Here's how the part is built. I have some questions about the finished solid (model axes, mm). A direction names the side the tool comes from. Coordinates: 2 decimals unless noted, no trailing zeros. Loops run counter-clockwise (first coordinate to the right, second up) from the corner with the lowest first, then second, coordinate; pieces in that order, holes last. Notation, with made-up numbers: (-23, 43.5) -> (-18, 43.5) arc R15 cw to (-18, 71.5) -> close; hole circle Ø5 at (6, 71.25). An arc over 180 degrees is marked (long way). Answer as a JSON object with one key per item and string values. Group by question number.
Q1. I want a section at A-A on z = -129. Write out the boundary of the cut face in (x, y).
Q2. I'm going to push flat-ended pins straight in: pin 1 (2 mm diameter, centred on x = -23, z = -92.5, fed in from -Y); pin 2 (12 mm diameter, centred on y = 8, z = -45, fed in from -X); pin 3 (1 mm diameter, centred on x = 4, z = -14.5, fed in from -Y). Where does each tip first touch, or does it pass through?
Q3. I need wall thicknesses on line 1 (Z direction, x = 36.5, y = 57); line 2 (Z direction, x = -36, y = 43.5); line 3 (X direction, y = -35, z = -122). Which ranges of each line are inside material? Lowest first, please.
Q4. I want a section at B-B on z = -12. Write out the boundary of the cut face in (x, y).
Q5. Thinking about a two-plate mould opening in Y: for faces 3 (the flat face through (0, 0, 47.5)), 4 (the conical face through (6.068, 46.217, -59.383)), which applies, released by +Y, released by -Y, zero draft, split by the parting line, or undercut?
Q6. On a 3-axis mill with a long thin cutter (end or side, diameter ignored), from which of +Z, -Z, +X, -X, +Y, -Y can I reach the whole of each face in a straight line? I mean faces 1 (the flat face through (1, 1, -150)), 2 (the cylindrical face through (12.365, -19.394, 3.014)). Say none if no direction works.
```python
from build123d import *

# Parameters (mm, degrees)
FILLET1_R = 10


with BuildPart() as part:
    # Sketch1 → Revolve1 (revolve)
    with BuildSketch(Plane.YZ, mode=Mode.PRIVATE) as revolve1_sk:
        with BuildLine():
            Line((0, 0), (-25, 0))
            Line((-25, 0), (-25, 2))
            Line((-25, 2), (-23, 2))
            Line((-23, 2), (-23, 4))
            ThreePointArc((-23, 4), (-19.907119135, 18.74298562), (-11.15, 31))
            Line((-11.15, 31), (-11.15, 47.5))
            Line((-11.15, 47.5), (0, 47.5))
            Line((0, 47.5), (0, 0))
        make_face()
    revolve(revolve1_sk.sketch.rotate(Axis((0, 0, 47.5), (0, 0, -1)), 270), axis=Axis((0, 0, 47.5), (0, 0, -1)))

    # Fillet1
    fillet1_edges = [part.edges().sort_by_distance(p)[0] for p in [
        (-11.15, 0, 31),
    ]]
    fillet(fillet1_edges, radius=FILLET1_R)

    # Sketch2 → Revolve2 (revolve)
    with BuildSketch(Plane.YZ, mode=Mode.PRIVATE) as revolve2_sk:
        Polygon((-25, 0), (-79.59553514, -150), (0, -150), (0, 0), align=None)
    revolve(revolve2_sk.sketch.rotate(Axis((0, 0, 0), (0, 0, -1)), 90), axis=Axis((0, 0, 0), (0, 0, -1)))


solid = part.part
```
Result set:
{
 "1": {"outline": "circle Ø143.9 at (0, 0)"},
 "2": {"pin 1": "stops at y = -54.54", "pin 2": "stops at x = -43.02", "pin 3": "stops at y = -30.21"},
 "3": {"line 1": "z = -150 to -117.28", "line 2": "z = -150 to -86.45", "line 3": "x = -59.93 to 59.93"},
 "4": {"outline": "circle Ø58.74 at (0, 0)"},
 "5": {"face 3": "zero draft", "face 4": "split by the parting line"},
 "6": {"face 1": "-Z, +X, -X, +Y, -Y", "face 2": "+Z"}
}
